```python
from build123d import *

# Parameters (mm, degrees)
BOSS_EXTRUDE1_DEPTH     = 8
BOSS_EXTRUDE2_START     = 8
SKETCH1_4_W             = 10.4
SKETCH1_4_H             = 12.4
BOSS_EXTRUDE2_DEPTH     = 24.8
CUT_EXTRUDE3_DEPTH      = 177.890212798
CUT_EXTRUDE3_DEPTH_BACK = 182.890212798
CUT_EXTRUDE3_START      = 5
SKETCH1_6_W             = 10.4
SKETCH1_6_H             = 12.4
SKETCH1_6_R             = 1.7
BOSS_EXTRUDE3_START     = -16.8
SKETCH1_10_W            = 11.4
SKETCH1_10_H            = 13.4
SKETCH1_10_W_2          = 10.4
SKETCH1_10_H_2          = 12.4
SKETCH1_10_W_3          = 7
SKETCH1_10_H_3          = 9
BOSS_EXTRUDE3_DEPTH     = 0.7
SKETCH2_R               = 1.7
SKETCH2_W               = 10.4
SKETCH2_H               = 12.4
CUT_EXTRUDE7_DEPTH      = 3
CUT_EXTRUDE5_START      = 8
SKETCH1_8_R             = 1.7
CUT_EXTRUDE5_DEPTH      = 3
CUT_EXTRUDE6_DEPTH      = 3


with BuildPart() as part:
    # Sketch1 → Boss-Extrude1 (new body)
    with BuildSketch(Plane(origin=(0, 0, 0), x_dir=(1, 0, 0), z_dir=(0, 1, 0))):
        with BuildLine():
            Line((-15.556349186, 15.556349186), (90.509667992, 121.622366364))
            ThreePointArc((90.509667992, 121.622366364), (121.622366364, 121.622366364), (121.622366364, 90.509667992))
            Line((121.622366364, 90.509667992), (15.556349186, -15.556349186))
            ThreePointArc((15.556349186, -15.556349186), (-15.556349186, -15.556349186), (-15.556349186, 15.556349186))
        make_face()
    extrude(amount=BOSS_EXTRUDE1_DEPTH)

    # Sketch1<4> → Boss-Extrude2 (add)
    with BuildSketch(Plane(origin=(0, 0, 0), x_dir=(1, 0, 0), z_dir=(0, 1, 0)).offset(BOSS_EXTRUDE2_START)):
        with BuildLine():
            ThreePointArc((-5.7, 6.7), (0, 10.065795515), (5.7, 6.7))
            ThreePointArc((5.7, 6.7), (7.425074212, 0), (5.7, -6.7))
            ThreePointArc((5.7, -6.7), (0, -10.065795515), (-5.7, -6.7))
            ThreePointArc((-5.7, -6.7), (-7.425074212, 0), (-5.7, 6.7))
        make_face()
        Rectangle(SKETCH1_4_W, SKETCH1_4_H, mode=Mode.SUBTRACT)
    extrude(amount=-BOSS_EXTRUDE2_DEPTH)

    # Sketch1<6> → Cut-Extrude3 (cut, two sides: drawn at the far end of the back side and taken through both)
    with BuildSketch(Plane(origin=(0, 0, 0), x_dir=(1, 0, 0), z_dir=(0, 1, 0)).offset(CUT_EXTRUDE3_START - CUT_EXTRUDE3_DEPTH_BACK)):
        Rectangle(SKETCH1_6_W, SKETCH1_6_H)
        with Locations(Location((106.066017178, 106.066017178, 0), (0, 0, 270))):
            Circle(SKETCH1_6_R)
        with Locations(Location((99.718863875, 119.666151183, 0), (0, 0, 270))):
            Circle(SKETCH1_6_R)
        with Locations(Location((91.11521733, 107.378870518, 0), (0, 0, 270))):
            Circle(SKETCH1_6_R)
        with Locations(Location((11, 0, 0), (0, 0, 270))):
            Circle(SKETCH1_6_R)
        with Locations(Location((-11, 0, 0), (0, 0, 270))):
            Circle(SKETCH1_6_R)
    extrude(amount=CUT_EXTRUDE3_DEPTH + CUT_EXTRUDE3_DEPTH_BACK, mode=Mode.SUBTRACT)

    # Sketch1<10> → Boss-Extrude3 (add)
    # profile 1 of 6: a face of its own
    with BuildSketch(Plane(origin=(0, 0, 0), x_dir=(1, 0, 0), z_dir=(0, 1, 0)).offset(BOSS_EXTRUDE3_START)):
        Rectangle(SKETCH1_10_W, SKETCH1_10_H)
        Rectangle(SKETCH1_10_W_2, SKETCH1_10_H_2, mode=Mode.SUBTRACT)
    # profile 2 of 6: a face of its own
    with BuildSketch(Plane(origin=(0, 0, 0), x_dir=(1, 0, 0), z_dir=(0, 1, 0)).offset(BOSS_EXTRUDE3_START)):
        Rectangle(SKETCH1_10_W_2, SKETCH1_10_H_2)
        Rectangle(SKETCH1_10_W_3, SKETCH1_10_H_3, mode=Mode.SUBTRACT)
    # profile 3 of 6: a face of its own
    with BuildSketch(Plane(origin=(0, 0, 0), x_dir=(1, 0, 0), z_dir=(0, 1, 0)).offset(BOSS_EXTRUDE3_START)):
        with BuildLine():
            ThreePointArc((-5.7, 6.7), (0, 10.065795515), (5.7, 6.7))
            Line((5.7, 6.7), (-5.7, 6.7))
        make_face()
    # profile 4 of 6: a face of its own
    with BuildSketch(Plane(origin=(0, 0, 0), x_dir=(1, 0, 0), z_dir=(0, 1, 0)).offset(BOSS_EXTRUDE3_START)):
        with BuildLine():
            Line((5.7, 6.7), (5.7, -6.7))
            ThreePointArc((5.7, -6.7), (7.425074212, 0), (5.7, 6.7))
        make_face()
    # profile 5 of 6: a face of its own
    with BuildSketch(Plane(origin=(0, 0, 0), x_dir=(1, 0, 0), z_dir=(0, 1, 0)).offset(BOSS_EXTRUDE3_START)):
        with BuildLine():
            Line((-5.7, -6.7), (5.7, -6.7))
            ThreePointArc((5.7, -6.7), (0, -10.065795515), (-5.7, -6.7))
        make_face()
    # profile 6 of 6: a face of its own
    with BuildSketch(Plane(origin=(0, 0, 0), x_dir=(1, 0, 0), z_dir=(0, 1, 0)).offset(BOSS_EXTRUDE3_START)):
        with BuildLine():
            Line((-5.7, 6.7), (-5.7, -6.7))
            ThreePointArc((-5.7, -6.7), (-7.425074212, 0), (-5.7, 6.7))
        make_face()
    extrude(amount=-BOSS_EXTRUDE3_DEPTH)

    # Sketch2 → Cut-Extrude7 (cut)
    with BuildSketch(Plane(origin=(0, 8, 0), x_dir=(1, 0, 0), z_dir=(0, 1, 0))):
        with BuildLine():
            ThreePointArc((-3.784090909, -8.440566094), (0, -9.25), (3.784090909, -8.440566094))
            Line((3.784090909, -8.440566094), (12.943181818, -4.334344751))
            ThreePointArc((12.943181818, -4.334344751), (15.75, 0), (12.943181818, 4.334344751))
            Line((12.943181818, 4.334344751), (3.784090909, 8.440566094))
            ThreePointArc((3.784090909, 8.440566094), (0, 9.25), (-3.784090909, 8.440566094))
            Line((-3.784090909, 8.440566094), (-12.943181818, 4.334344751))
            ThreePointArc((-12.943181818, 4.334344751), (-15.75, 0), (-12.943181818, -4.334344751))
            Line((-12.943181818, -4.334344751), (-3.784090909, -8.440566094))
        make_face()
        with Locations(Location((-11, 0, 0), (0, 0, 270))):
            Circle(SKETCH2_R, mode=Mode.SUBTRACT)
        Rectangle(SKETCH2_W, SKETCH2_H, mode=Mode.SUBTRACT)
        with Locations(Location((11, 0, 0), (0, 0, 270))):
            Circle(SKETCH2_R, mode=Mode.SUBTRACT)
    extrude(amount=-CUT_EXTRUDE7_DEPTH, mode=Mode.SUBTRACT)

    # Sketch1<8> → Cut-Extrude5 (cut)
    # profile 1 of 3: a face of its own
    with BuildSketch(Plane(origin=(0, 0, 0), x_dir=(1, 0, 0), z_dir=(0, 1, 0)).offset(CUT_EXTRUDE5_START)):
        Polygon((102.168353618, 117.21666144), (103.06492909, 120.562726655), (100.615439347, 123.012216398), (97.269374132, 122.115640925), (96.37279866, 118.769575711), (98.822288403, 116.320085968), align=None)
        with Locations(Location((99.718863875, 119.666151183, 0), (0, 0, 270))):
            Circle(SKETCH1_8_R, mode=Mode.SUBTRACT)
    # profile 2 of 3: a face of its own
    with BuildSketch(Plane(origin=(0, 0, 0), x_dir=(1, 0, 0), z_dir=(0, 1, 0)).offset(CUT_EXTRUDE5_START)):
        Polygon((88.665727587, 109.828360261), (87.769152115, 106.482295046), (90.218641857, 104.032805303), (93.564707072, 104.929380776), (94.461282545, 108.275445991), (92.011792802, 110.724935733), align=None)
        with Locations(Location((91.11521733, 107.378870518, 0), (0, 0, 270))):
            Circle(SKETCH1_8_R, mode=Mode.SUBTRACT)
    # profile 3 of 3: a face of its own
    with BuildSketch(Plane(origin=(0, 0, 0), x_dir=(1, 0, 0), z_dir=(0, 1, 0)).offset(CUT_EXTRUDE5_START)):
        Polygon((108.515506921, 103.616527435), (109.412082393, 106.96259265), (106.96259265, 109.412082393), (103.616527435, 108.515506921), (102.719951963, 105.169441706), (105.169441706, 102.719951963), align=None)
        with Locations(Location((106.066017178, 106.066017178, 0), (0, 0, 270))):
            Circle(SKETCH1_8_R, mode=Mode.SUBTRACT)
    extrude(amount=-CUT_EXTRUDE5_DEPTH, mode=Mode.SUBTRACT)

    # Sketch1<9> → Cut-Extrude6 (cut)
    with BuildSketch(Plane(origin=(0, 0, 0), x_dir=(1, 0, 0), z_dir=(0, 1, 0))):
        with BuildLine():
            Line((97.232940058, 93.451075696), (-9.918409797, 168.479258594))
            ThreePointArc((-9.918409797, 168.479258594), (-13.700274159, 189.927277196), (7.747744443, 193.709141558))
            Line((7.747744443, 193.709141558), (114.899094298, 118.68095866))
            ThreePointArc((114.899094298, 118.68095866), (118.68095866, 97.232940058), (97.232940058, 93.451075696))
        make_face()
    extrude(amount=CUT_EXTRUDE6_DEPTH, mode=Mode.SUBTRACT)


solid = part.part
```
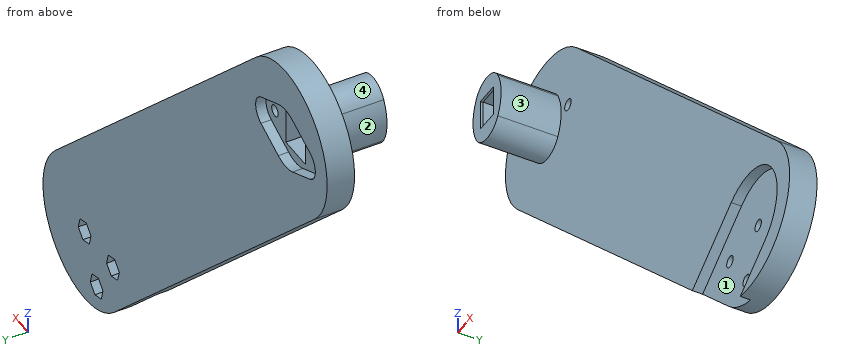
The model under review builds one solid part; all positions refer to its coordinate system, in mm. Face numbers are marked on the shaded views. A direction names the side the tool comes from. Round coordinates to 2 decimals unless told otherwise and drop trailing zeros. Loops run counter-clockwise (first coordinate to the right, second up) from the corner with the lowest first, then second, coordinate; pieces in that order, holes last. Notation, with made-up numbers: (48.25, 77.5) -> (79.25, 77.5) arc R10 ccw to (79.25, 87.5) -> close; hole circle Ø7 at (15.5, 70.5). An arc over 180 degrees is marked (long way). Answer as a JSON object with one key per item and string values. Group by question number.
1) We need section A-A on y = -3.5. Write out the cut boundary in (x, z), then the cut area to 3 significant figures.
2) We need section B-B on x = 118. Write out the cut boundary in (y, z).
3) We need section D-D on x = 35. Write out the cut boundary in (y, z), then the cut area to 3 significant figures.
4) For line 1 (X direction, y = 2.4, z = 0); line 2 (Y direction, x = 26, z = -39); line 3 (Z direction, x = 11, y = 2.75), list the stretches that pass through material, from the lowest coordinate up. Write a range as [from, to].
5) We need section C-C on z = -58.5. Write out the cut boundary in (x, y).
6) For the marked faces 1, 2, 3 and 4, list the 3-axis set-ups (+Z, -Z, +X, -X, +Y, -Y) from which the entire face can be reached by the end or side of a thin tool; tool diameter is ignored.
7) For pin 1 Ø0.6 at (y, z) = (-17, 1) entering from -X; pin 2 Ø2 at (x, z) = (99.5, -121) entering from +Y; pin 3 Ø8.5 at (x, y) = (2.5, -5) entering from +Z; pin 4 Ø2.5 at (x, z) = (91.12, -107.38) entering from -Y, all flat-tipped, find the tip position at first contact; note any pin that passes through.
Result set:
{
 "1": {"outline": "(-5.7, -6.7) arc R6.51 ccw to (5.7, -6.7) arc R13.87 ccw to (5.7, 6.7) arc R6.51 ccw to (-5.7, 6.7) arc R13.87 ccw to start; hole (-5.2, -6.2) -> (5.2, -6.2) -> (5.2, 6.2) -> (-5.2, 6.2) -> close", "area": "110 mm²"},
 "2": {"outline": "(0, -124.55) -> (8, -124.55) -> (8, -86.89) -> (0, -86.89) -> (0, -96.33) -> (3, -96.33) -> (3, -115.8) -> (0, -115.8) -> close"},
 "3": {"outline": "(0, -66.11) -> (8, -66.11) -> (8, -3.89) -> (0, -3.89) -> close", "area": "498 mm²"},
 "4": {"line 1": "[-22, -12.7], [-9.3, -5.2], [5.2, 9.3], [12.7, 31.11]", "line 2": "[0, 8]", "line 3": "[-42.11, -1.7], [1.7, 19.05]"},
 "5": {"outline": "(27.39, 0) -> (89.61, 0) -> (89.61, 8) -> (27.39, 8) -> close"},
 "6": {"face 1": "-Y", "face 2": "-X, -Y", "face 3": "+X, -Y", "face 4": "+Z, -Y"},
 "7": {"pin 1": "x = -7.41", "pin 2": "y = 5", "pin 3": "z = 10.07", "pin 4": "through"}
}
